Study the drawing (mm; zero at the part's minimum x, y, z) and answer. Round coordinates to 2 decimals unless told otherwise and drop trailing zeros. Write each loop counter-clockwise with the first axis right and the second up, starting at its lowest first coordinate (ties: lowest second). Pieces come first, ordered by that corner, then holes.
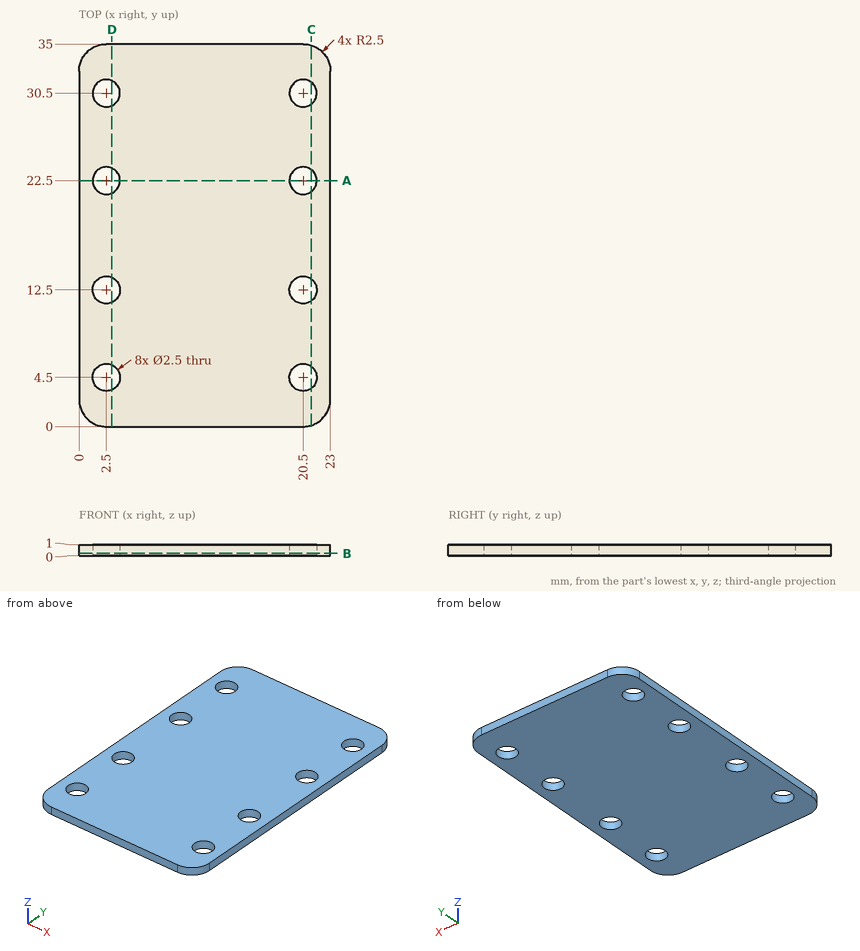
1. Section A-A on y = 22.5 is taken. Determine the outline of the cut face in (x, z).
Geometry says:
outline: (0, 0) - (1.25, 0) - (1.25, 1) - (0, 1) - close; (3.75, 0) - (19.25, 0) - (19.25, 1) - (3.75, 1) - close; (21.75, 0) - (23, 0) - (23, 1) - (21.75, 1) - close
2. Given pin 1 (3 mm diameter, centred on x = 20.5, y = 30.5, fed in from -Z), flat-ended and moving along its own axis, determine where the tip first touches the part or whether it passes through.
Geometry says:
pin 1: stops at z = 0
3. Straight lines are drawn through the part: line 1 along Y through (x, z) = (2.5, 0.55); line 2 along X through (y, z) = (30.5, 0.5); line 3 along Y through (x, z) = (19.75, 0.15). For each, find the intervals that lie inside material, in ascending order.
Geometry says:
line 1: y = 0 to 3.25, 5.75 to 11.25, 13.75 to 21.25, 23.75 to 29.25, 31.75 to 35
line 2: x = 0 to 1.25, 3.75 to 19.25, 21.75 to 23
line 3: y = 0 to 3.5, 5.5 to 11.5, 13.5 to 21.5, 23.5 to 29.5, 31.5 to 35
4. Section B-B on z = 0.2 is taken. Give the number of separate pieces and of enclosed holes in the cut face, plus the area to 3 significant figures.
Geometry says:
separate pieces: 1
enclosed holes: 8
area: 760 mm2
5. Section C-C on x = 21.25 is taken. Determine the outline of the cut face in (y, z), plus the area to 3 significant figures.
Geometry says:
outline: (0.12, 0) - (3.5, 0) - (3.5, 1) - (0.12, 1) - close; (5.5, 0) - (11.5, 0) - (11.5, 1) - (5.5, 1) - close; (13.5, 0) - (21.5, 0) - (21.5, 1) - (13.5, 1) - close; (23.5, 0) - (29.5, 0) - (29.5, 1) - (23.5, 1) - close; (31.5, 0) - (34.88, 0) - (34.88, 1) - (31.5, 1) - close
area: 26.8 mm2
6. Section D-D on x = 3 is taken. Determine the outline of the cut face in (y, z), plus the area to 3 significant figures.
Geometry says:
outline: (0, 0) - (3.35, 0) - (3.35, 1) - (0, 1) - close; (5.65, 0) - (11.35, 0) - (11.35, 1) - (5.65, 1) - close; (13.65, 0) - (21.35, 0) - (21.35, 1) - (13.65, 1) - close; (23.65, 0) - (29.35, 0) - (29.35, 1) - (23.65, 1) - close; (31.65, 0) - (35, 0) - (35, 1) - (31.65, 1) - close
area: 25.8 mm2
